Geometry: final body of the model. Coordinates: model frame, mm. Round coordinates to 2 decimals unless told otherwise and drop trailing zeros. Loops run counter-clockwise (first coordinate to the right, second up) from the corner with the lowest first, then second, coordinate; pieces in that order, holes last. Notation, with made-up numbers: M 0.25,89.25 L 44.25,89.25 A32 cw 44.25,124.25 Z; hole C -14,19 d10. An arc over 180 degrees is marked long. Answer as a JSON object with one key per item and string values.
```python
from build123d import *

# Parameters (mm, degrees)
SKETCH_R    = 1.75
SKETCH_W    = 6
SKETCH_H    = 15
PAD_DEPTH   = 3
FILLET_R    = 3
FILLET001_R = 1


with BuildPart() as part:
    # Sketch → Pad (new body)
    with BuildSketch(Plane.XY):
        Polygon((25.05, 23), (39.95, 23), (39.95, 20), (70.05, 20), (70.05, 23), (84.95, 23), (84.95, 20), (103.7, 20), (103.7, -20), (84.95, -20), (84.95, -23), (70.05, -23), (70.05, -20), (39.95, -20), (39.95, -23), (25.05, -23), (25.05, -20), (-25.05, -20), (-25.05, -23), (-39.95, -23), (-39.95, -20), (-70.05, -20), (-70.05, -23), (-84.95, -23), (-84.95, -20), (-103.7, -20), (-103.7, 20), (-84.95, 20), (-84.95, 23), (-70.05, 23), (-70.05, 20), (-39.95, 20), (-39.95, 23), (-25.05, 23), (-25.05, 20), (25.05, 20), align=None)
        with Locations((-70, 10)):
            Circle(SKETCH_R, mode=Mode.SUBTRACT)
        with Locations((-60, 10)):
            Circle(SKETCH_R, mode=Mode.SUBTRACT)
        with Locations((-70, -10)):
            Circle(SKETCH_R, mode=Mode.SUBTRACT)
        with Locations((-60, -10)):
            Circle(SKETCH_R, mode=Mode.SUBTRACT)
        with Locations((-50.463539, 0)):
            Rectangle(SKETCH_W, SKETCH_H, mode=Mode.SUBTRACT)
    extrude(amount=PAD_DEPTH)

    # Fillet
    fillet_edges = [part.edges().sort_by_distance(p)[0] for p in [
        (-103.7, 20, 1.5),
        (103.7, 20, 1.5),
        (103.7, -20, 1.5),
        (-103.7, -20, 1.5),
    ]]
    fillet(fillet_edges, radius=FILLET_R)

    # Fillet001
    fillet001_edges = [part.edges().sort_by_distance(p)[0] for p in [
        (-84.95, 23, 1.5),
        (-70.05, 23, 1.5),
        (-84.95, -23, 1.5),
        (-39.95, 23, 1.5),
        (-70.05, -23, 1.5),
        (-25.05, 23, 1.5),
        (-39.95, -23, 1.5),
        (25.05, 23, 1.5),
        (-25.05, -23, 1.5),
        (39.95, 23, 1.5),
        (25.05, -23, 1.5),
        (70.05, 23, 1.5),
        (39.95, -23, 1.5),
        (84.95, 23, 1.5),
        (70.05, -23, 1.5),
        (84.95, -23, 1.5),
        (-53.463539, -7.5, 1.5),
        (-53.463539, 7.5, 1.5),
        (-47.463539, -7.5, 1.5),
        (-47.463539, 7.5, 1.5),
    ]]
    fillet(fillet001_edges, radius=FILLET001_R)


solid = part.part
```
1) Cut plane C-C on y = -10. Return the cut outline in (x, z), and give its area (3 significant figures).
Geometry results:
{"outline": "M -103.7,0 L -71.75,0 L -71.75,3 L -103.7,3 Z; M -68.25,0 L -61.75,0 L -61.75,3 L -68.25,3 Z; M -58.25,0 L 103.7,0 L 103.7,3 L -58.25,3 Z", "area": "601 mm2"}
2) Line query: probe 1 along X at (y, z) = (20.5, 2.6); probe 2 along Y at (x, z) = (-70, 1.65); probe 3 along X at (y, z) = (-3, 1.6). Output: solid intervals per line, ascending.
Geometry results:
{"probe 1": "-84.95 to -70.05, -39.95 to -25.05, 25.05 to 39.95, 70.05 to 84.95", "probe 2": "-20 to -11.75, -8.25 to 8.25, 11.75 to 20", "probe 3": "-103.7 to -53.46, -47.46 to 103.7"}
3) Cut plane D-D on z = 2.05. Count the separate pieces of the cut face and the enclosed holes in it, and give its area (3 significant figures).
Geometry results:
{"separate pieces": "1", "enclosed holes": "5", "area": "8,510 mm2"}
4) First-contact query: pin 1 (1.6 mm diameter, centred on y = 20.5, z = 2, fed in from +X); pin 2 (1.5 mm diameter, centred on x = 63, z = 1.5, fed in from -Y); pin 3 (1 mm diameter, centred on y = -21.5, z = 2, fed in from +X). Flat tips, straight axial feed; report the tip coordinate or a pass-through.
Geometry results:
{"pin 1": "x = 102.01", "pin 2": "y = -20", "pin 3": "x = 84.95"}
5) Cut plane B-B on x = -60. Return the cut outline in (y, z).
Geometry results:
{"outline": "M -20,0 L -11.75,0 L -11.75,3 L -20,3 Z; M -8.25,0 L 8.25,0 L 8.25,3 L -8.25,3 Z; M 11.75,0 L 20,0 L 20,3 L 11.75,3 Z"}
6) Cut plane A-A on y = -1.5. Return the cut outline in (x, z).
Geometry results:
{"outline": "M -103.7,0 L -53.46,0 L -53.46,3 L -103.7,3 Z; M -47.46,0 L 103.7,0 L 103.7,3 L -47.46,3 Z"}
7) Pull-direction query (Y, two-part tool) for faces 1 (the face through (1, 0, 3)), 2 (the face through (-68.331, 10.526, 1.479)); classes: +Y half, -Y half, draft (parallel to the pull), parting line (faces both ways), or undercut.
Geometry results:
{"face 1": "draft", "face 2": "undercut"}
